```python
from build123d import *

# Parameters (mm, degrees)
SKETCH_1_R      = 1.55
SKETCH_1_R_2    = 1.3
SKETCH_1_R_3    = 12
EXTRUDE_1_DEPTH = 2
SKETCH_2_W      = 5.700941524
SKETCH_2_H      = 9
SKETCH_2_R      = 1.3
EXTRUDE_2_DEPTH = 3


with BuildPart() as part:
    # 草图1 → 凸台-拉伸1 (new body)
    with BuildSketch(Plane.XY):
        Polygon((118, -35), (118, 35), (5, 35), (5, 19), (5, -17), (-7.054941738, -17), (-7.054941738, 4.999698131), (-7.054941738, 11.999849066), (-30, 11.999849066), (-30, -35), (-7.054941738, -35), (17.9, -35), align=None)
        with Locations((-25, -24)):
            Circle(SKETCH_1_R, mode=Mode.SUBTRACT)
        with Locations((-15, -24)):
            Circle(SKETCH_1_R, mode=Mode.SUBTRACT)
        with Locations((10, -25)):
            Circle(SKETCH_1_R, mode=Mode.SUBTRACT)
        with Locations((-25, -5)):
            Circle(SKETCH_1_R, mode=Mode.SUBTRACT)
        with Locations((-15, -5)):
            Circle(SKETCH_1_R, mode=Mode.SUBTRACT)
        with Locations((60, -25)):
            Circle(SKETCH_1_R_2, mode=Mode.SUBTRACT)
        with Locations((90, -30)):
            Circle(SKETCH_1_R, mode=Mode.SUBTRACT)
        with Locations((100, -25)):
            Circle(SKETCH_1_R_2, mode=Mode.SUBTRACT)
        with Locations((110, -20)):
            Circle(SKETCH_1_R, mode=Mode.SUBTRACT)
        with Locations((-25, 5)):
            Circle(SKETCH_1_R, mode=Mode.SUBTRACT)
        with Locations((-15.054941738, 4.999698131)):
            Circle(SKETCH_1_R, mode=Mode.SUBTRACT)
        with Locations((10, 9.1)):
            Circle(SKETCH_1_R, mode=Mode.SUBTRACT)
        with Locations((19.9, 9.1)):
            Circle(SKETCH_1_R, mode=Mode.SUBTRACT)
        with Locations((39.7, 9.1)):
            Circle(SKETCH_1_R, mode=Mode.SUBTRACT)
        with Locations((10, 19)):
            Circle(SKETCH_1_R, mode=Mode.SUBTRACT)
        with Locations((19.9, 19)):
            Circle(SKETCH_1_R, mode=Mode.SUBTRACT)
        with Locations((39.7, 19)):
            Circle(SKETCH_1_R, mode=Mode.SUBTRACT)
        with Locations((100, 0)):
            Circle(SKETCH_1_R_3, mode=Mode.SUBTRACT)
        with Locations((60, 25)):
            Circle(SKETCH_1_R_2, mode=Mode.SUBTRACT)
        with Locations((110, 20)):
            Circle(SKETCH_1_R, mode=Mode.SUBTRACT)
        with Locations((100, 25)):
            Circle(SKETCH_1_R_2, mode=Mode.SUBTRACT)
        with Locations((90, 30)):
            Circle(SKETCH_1_R, mode=Mode.SUBTRACT)
    extrude(amount=EXTRUDE_1_DEPTH)

    # 草图2 → 凸台-拉伸2 (add)
    with BuildSketch(Plane(origin=(0, 0, 0), x_dir=(-1, 0, 0), z_dir=(0, 0, -1))):
        Polygon((-62.898115349, 2.499732073), (-57.197173825, 9), (-34.39434765, 35), (-44.39434765, 35), (-55.898115349, 21.883294295), (-57.635924693, 19.901827498), (-62.898115349, 13.901827498), (-90, -17), (-80, -17), align=None)
        Polygon((30, -21), (30, -17), (7.054941738, -17), (-5, -17), (-57.197173825, -17), (-62.898115349, -17), (-80, -17), (-90, -17), (-90, -21), (-62.898115349, -21), (-57.197173825, -21), align=None)
        Polygon((30, -35), (30, -30), (-57.197173825, -30), (-62.898115349, -30), (-80, -30), (-80, -35), align=None)
        Polygon((-101.707321844, 13.901827498), (-62.898115349, 13.901827498), (-57.635924693, 19.901827498), (-62.898115349, 19.901827498), (-101.707321844, 19.901827498), align=None)
        with Locations((-60.047644587, -25.5)):
            Rectangle(SKETCH_2_W, SKETCH_2_H)
        with Locations((-60, -25)):
            Circle(SKETCH_2_R, mode=Mode.SUBTRACT)
        Polygon((-62.898115349, -17), (-57.197173825, -17), (-57.197173825, 9), (-62.898115349, 2.499732073), align=None)
        Polygon((-57.635924693, 19.901827498), (-55.898115349, 21.883294295), (-55.898115349, 35), (-62.898115349, 35), (-62.898115349, 19.901827498), align=None)
        with Locations((-60, 25)):
            Circle(SKETCH_2_R, mode=Mode.SUBTRACT)
    extrude(amount=EXTRUDE_2_DEPTH)


solid = part.part
```
The listing builds one solid part. Answer for the finished solid, in the listing's coordinates (mm). A direction names the side the tool comes from. Give positions to 0.01 mm unless a question says otherwise; leave off trailing zeros. Write each loop counter-clockwise with the first axis right and the second up, starting at its lowest first coordinate (ties: lowest second). Pieces come first, ordered by that corner, then holes. Notation, with made-up numbers: (46.25, -12.5) -> (53.25, -12.5) arc R17 cw to (53.25, -1.5) -> close; hole circle Ø3 at (56.25, 38.5). An arc over 180 degrees is marked (long way). Use one line per item in the form item = value.
1) Section B-B on z = -1.4 is taken. Write down the section's boundary in (x, y).
Result:
outline = (-30, -35) -> (80, -35) -> (80, -30) -> (62.9, -30) -> (62.9, -21) -> (90, -21) -> (90, -17) -> (62.9, 13.9) -> (101.71, 13.9) -> (101.71, 19.9) -> (62.9, 19.9) -> (62.9, 35) -> (55.9, 35) -> (55.9, 21.88) -> (44.39, 35) -> (34.39, 35) -> (57.2, 9) -> (57.2, -17) -> (-30, -17) -> (-30, -21) -> (57.2, -21) -> (57.2, -30) -> (-30, -30) -> close; hole circle Ø2.6 at (60, -25); hole circle Ø2.6 at (60, 25); hole (62.9, -17) -> (80, -17) -> (62.9, 2.5) -> close
2) Section A-A on x = 10 is taken. Write down the section's boundary in (y, z), plus the area to 3 significant figures.
Result:
outline = (-35, -3) -> (-30, -3) -> (-30, 0) -> (-26.55, 0) -> (-26.55, 2) -> (-35, 2) -> close; (-23.45, 0) -> (-21, 0) -> (-21, -3) -> (-17, -3) -> (-17, 0) -> (7.55, 0) -> (7.55, 2) -> (-23.45, 2) -> close; (10.65, 0) -> (17.45, 0) -> (17.45, 2) -> (10.65, 2) -> close; (20.55, 0) -> (35, 0) -> (35, 2) -> (20.55, 2) -> close
area = 148 mm²
3) Section C-C on y = 30 is taken. Write down the section's boundary in (x, z).
Result:
outline = (5, 0) -> (38.78, 0) -> (38.78, -3) -> (48.78, -3) -> (48.78, 0) -> (55.9, 0) -> (55.9, -3) -> (62.9, -3) -> (62.9, 0) -> (88.45, 0) -> (88.45, 2) -> (5, 2) -> close; (91.55, 0) -> (118, 0) -> (118, 2) -> (91.55, 2) -> close
4) For a pull along X with two mould halves and no side action, classify faces 1 (the flat face through (62.898, 28, -1)), 2 (the cylindrical face through (-23.568, 4.406, 0.986)), 3 (the flat face through (71, -30, -1)) as +X half, -X half, draft (parallel to the pull), parting line (faces both ways), or undercut.
Result:
face_1 = +X half
face_2 = undercut
face_3 = draft
5) Each of these flat-tipped pins is pushed along its axis until it touches: P1, Ø3, axis at y = 17.5, z = 0, coming from the -X side; P2, Ø1.5, axis at x = 69, z = -2, coming from the +Y side; P3, Ø1.5, axis at y = -7.5, z = -2, coming from the -X side. Where does it stop, or does it pass through?
Result:
P1 = 5
P2 = 19.9
P3 = 57.2
6) Straight lines are drawn through the part: probe 1 along Y at (x, z) = (-25, 1); probe 2 along X at (y, z) = (-0.5, 1.65); probe 3 along Y at (x, z) = (28.5, -2.65). For each, find the intervals that lie inside material, in ascending order.
Result:
probe_1 = -35 to -25.55, -22.45 to -6.55, -3.45 to 3.45, 6.55 to 12
probe_2 = -30 to -7.05, 5 to 88.01, 111.99 to 118
probe_3 = -35 to -30, -21 to -17
7) A tool of negligible diameter and unlimited length cuts with its end or side. For faces 4 (the flat face through (13, -25, 0)), 5 (the flat face through (71.57, -7.39, -1.48)), 6 (the flat face through (62.898, -26, -1)), from which of +Z, -Z, +X, -X, +Y, -Y can it reach the whole face along a straight path? Write none if from no direction.
Result:
face_4 = -Z, -X
face_5 = -Z
face_6 = -Z, +X
8) Section D-D on x = 50 is taken. Write down the section's boundary in (y, z), plus the area to 3 significant figures.
Result:
outline = (-35, -3) -> (-30, -3) -> (-30, 0) -> (-21, 0) -> (-21, -3) -> (-17, -3) -> (-17, 0) -> (17.21, 0) -> (17.21, -3) -> (28.61, -3) -> (28.61, 0) -> (35, 0) -> (35, 2) -> (-35, 2) -> close
area = 201 mm²
